```python
from build123d import *

# Parameters (mm, degrees)
SKETCH1_R           = 1.5
BOSS_EXTRUDE1_DEPTH = 6
SKETCH2_W           = 54
SKETCH2_H           = 3
BOSS_EXTRUDE2_DEPTH = 50
SKETCH4_R           = 1.5
SKETCH4_R_2         = 1
SKETCH4_W           = 12
SKETCH4_H           = 22.8
CUT_EXTRUDE1_DEPTH  = 24
SKETCH5_W           = 11
SKETCH5_H           = 4
CUT_EXTRUDE2_DEPTH  = 13.62
SKETCH6_R           = 1
CUT_EXTRUDE3_DEPTH  = 24
SKETCH7_R           = 1.5
CUT_EXTRUDE4_DEPTH  = 7
SKETCH8_R           = 1.5
CUT_EXTRUDE5_DEPTH  = 7
SKETCH3_R           = 1.5
CUT_EXTRUDE6_DEPTH  = 60
SKETCH9_R           = 1.5
CUT_EXTRUDE7_DEPTH  = 10


with BuildPart() as part:
    # Sketch1 → Boss-Extrude1 (new body)
    with BuildSketch(Plane.XY):
        Polygon((0, 0), (-4, 0), (-4, 20), (8, 20), (8, 33.5), (38, 33.5), (38, 20), (50, 20), (50, 0), (46, 0), (46, 17), (0, 17), align=None)
        with Locations((10.5, 26.75)):
            Circle(SKETCH1_R, mode=Mode.SUBTRACT)
        with Locations(Location((35.5, 26.75, 0), (0, 0, 180))):
            Circle(SKETCH1_R, mode=Mode.SUBTRACT)
    extrude(amount=BOSS_EXTRUDE1_DEPTH)

    # Sketch2 → Boss-Extrude2 (add)
    with BuildSketch(Plane.XY):
        with Locations((23, 18.5)):
            Rectangle(SKETCH2_W, SKETCH2_H)
    extrude(amount=BOSS_EXTRUDE2_DEPTH)

    # Sketch4 → Cut-Extrude1 (cut)
    with BuildSketch(Plane(origin=(0, 20, 0), x_dir=(1, 0, 0), z_dir=(0, 1, 0))):
        with Locations(Location((4.534048473, -3, 0), (0, 0, 270))):
            Circle(SKETCH4_R)
        with Locations(Location((1.5, -6.974235758, 0), (0, 0, 270))):
            Circle(SKETCH4_R)
        with Locations(Location((41.465951527, -3, 0), (0, 0, 180))):
            Circle(SKETCH4_R)
        with Locations(Location((44.5, -6.974235758, 0), (0, 0, 180))):
            Circle(SKETCH4_R)
        with Locations(Location((23, -31.8, 0), (0, 0, 270))):
            Circle(SKETCH4_R_2)
        with Locations((23, -17.4)):
            Rectangle(SKETCH4_W, SKETCH4_H)
    extrude(amount=-CUT_EXTRUDE1_DEPTH, mode=Mode.SUBTRACT)

    # Sketch5 → Cut-Extrude2 (cut)
    with BuildSketch(Plane(origin=(0, 33.5, 0), x_dir=(1, 0, 0), z_dir=(0, 1, 0))):
        with Locations((23, -4)):
            Rectangle(SKETCH5_W, SKETCH5_H)
    extrude(amount=-CUT_EXTRUDE2_DEPTH, mode=Mode.SUBTRACT)

    # Sketch6 → Cut-Extrude3 (cut)
    with BuildSketch(Plane(origin=(0, 19.88, 0), x_dir=(1, 0, 0), z_dir=(0, 1, 0))):
        with Locations(Location((23, -4, 0), (0, 0, 270))):
            Circle(SKETCH6_R)
    extrude(amount=-CUT_EXTRUDE3_DEPTH, mode=Mode.SUBTRACT)

    # Sketch7 → Cut-Extrude4 (cut)
    with BuildSketch(Plane.XZ):
        with Locations((48, 3)):
            Circle(SKETCH7_R)
    extrude(amount=-CUT_EXTRUDE4_DEPTH, mode=Mode.SUBTRACT)

    # Sketch8 → Cut-Extrude5 (cut)
    with BuildSketch(Plane.XZ):
        with Locations(Location((-2, 3, 0), (0, 0, 270))):
            Circle(SKETCH8_R)
    extrude(amount=-CUT_EXTRUDE5_DEPTH, mode=Mode.SUBTRACT)

    # Sketch3 → Cut-Extrude6 (cut)
    with BuildSketch(Plane(origin=(0, 20, 0), x_dir=(1, 0, 0), z_dir=(0, 1, 0))):
        with Locations(Location((0, -46, 0), (0, 0, 270))):
            Circle(SKETCH3_R)
        with Locations(Location((46, -46, 0), (0, 0, 270))):
            Circle(SKETCH3_R)
    extrude(amount=-CUT_EXTRUDE6_DEPTH, mode=Mode.SUBTRACT)

    # Sketch9 → Cut-Extrude7 (cut)
    with BuildSketch(Plane.XZ.offset(-17)):
        with Locations((48, 3)):
            Circle(SKETCH9_R)
        with Locations(Location((-2, 3, 0), (0, 0, 270))):
            Circle(SKETCH9_R)
    extrude(amount=-CUT_EXTRUDE7_DEPTH, mode=Mode.SUBTRACT)

    # SurfaceCut1
    split(bisect_by=Plane(origin=(0, 17, 0), x_dir=(-1, 0, 0), z_dir=(0, -1, 0)), keep=Keep.BOTTOM)


solid = part.part
```
Work out the finished part from the listing and answer in its coordinate system (mm). A direction names the side the tool comes from. Round coordinates to 2 decimals unless told otherwise and drop trailing zeros. Loops run counter-clockwise (first coordinate to the right, second up) from the corner with the lowest first, then second, coordinate; pieces in that order, holes last. Notation, with made-up numbers: (83.5, 87.25) -> (104.5, 87.25) arc R6 ccw to (104.5, 94.25) -> close; hole circle Ø3 at (36, 13.25). An arc over 180 degrees is marked (long way). Write each question's results on one line, items separated by ' | '. Start each with the question number.
1. Given pin 1 Ø3 at (y, z) = (24, 3.5) entering from -X; pin 2 Ø4 at (x, z) = (40.5, 23) entering from +Y, each flat-ended and moving along its own axis, determine where each tip first touches the part or whether it passes through.
2. Section B-B (z = 46) is taken. Determine the outline of the cut face in (x, y), plus the area to 3 significant figures.
3. For a pull along Y with two mould halves and no side action, classify faces 1 (the face through (36.61, 25.74, 2.96)), 2 (the face through (23, 17, 30)), 3 (the face through (23, 19, 28.8)) as +Y half, -Y half, draft (parallel to the pull), parting line (faces both ways), or undercut.
4. Section D-D (z = 31.8) is taken. Determine the outline of the cut face in (x, y), plus the area to 3 significant figures.
5. Section A-A (x = 20.5) is taken. Determine the outline of the cut face in (y, z).
6. A tool of negligible diameter and unlimited length cuts with its end or side. For faces 4 (the face through (17, 19, 18)), 5 (the face through (38, 27, 3)), 6 (the face through (17.5, 27, 4)), from which of +Z, -Z, +X, -X, +Y, -Y can it reach the whole face along a straight path? Write none if from no direction.
7. Section C-C (y = 26.75) is taken. Determine the outline of the cut face in (x, z).
8. Find the intervals of material crossed by probe 1 along Z at (x, y) = (18, 18.5); probe 2 along X at (y, z) = (17.85, 4); probe 3 along X at (y, z) = (19.35, 31.8), in increasing order. Write a range as from..to.
Evaluation:
1) pin 1: stops at x = 8 | pin 2: stops at y = 20
2) outline: (-4, 17) -> (-1.5, 17) -> (-1.5, 20) -> (-4, 20) -> close; (1.5, 17) -> (44.5, 17) -> (44.5, 20) -> (1.5, 20) -> close; (47.5, 17) -> (50, 17) -> (50, 20) -> (47.5, 20) -> close | area: 144 mm2
3) face 1: undercut | face 2: -Y half | face 3: draft
4) outline: (-4, 17) -> (22, 17) -> (22, 20) -> (-4, 20) -> close; (24, 17) -> (50, 17) -> (50, 20) -> (24, 20) -> close | area: 156 mm2
5) outline: (17, 0) -> (33.5, 0) -> (33.5, 2) -> (19.88, 2) -> (19.88, 6) -> (17, 6) -> close; (17, 28.8) -> (20, 28.8) -> (20, 50) -> (17, 50) -> close
6) face 4: +Y, -Y | face 5: +Z, -Z, +X, +Y | face 6: +Z, +Y
7) outline: (8, 0) -> (9, 0) -> (9, 6) -> (8, 6) -> close; (12, 0) -> (34, 0) -> (34, 6) -> (28.5, 6) -> (28.5, 2) -> (17.5, 2) -> (17.5, 6) -> (12, 6) -> close; (37, 0) -> (38, 0) -> (38, 6) -> (37, 6) -> close
8) probe 1: z = 0..6, 28.8..50 | probe 2: x = -4..-3.12, -0.88..3.42, 5.65..22, 24..40.35, 42.58..46.88, 49.12..50 | probe 3: x = -4..22, 24..50
